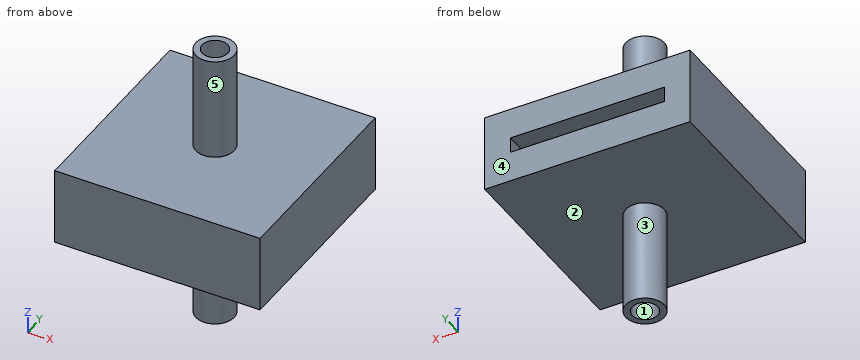
from build123d import *

# Parameters (mm, degrees)
F0_W      = 50.8
F0_H      = 50.8
F1_DEPTH  = 19.05
F2_W      = 38.1
F2_H      = 3.81
F3_DEPTH  = 38.1
F5_R      = 4.7625
F6_DEPTH  = 25.4
F7_R      = 4.7625
F8_DEPTH  = 25.4
F9_R      = 3.175
F10_DEPTH = 74.676


with BuildPart() as f1:
    # F0 (on Top) → F1 (new body)
    with BuildSketch(Plane.XY):
        Rectangle(F0_W, F0_H)
    extrude(amount=F1_DEPTH)

    # F2 (on face) → F3 (cut)
    with BuildSketch(Plane(origin=(0, 25.4, 0), x_dir=(-1, 0, 0), z_dir=(0, 1, 0))):
        with Locations((0, 9.525)):
            Rectangle(F2_W, F2_H)
    extrude(amount=-F3_DEPTH, mode=Mode.SUBTRACT)

    # F5 (on face) → F6 (join)
    with BuildSketch(Plane.XY.offset(19.05)):
        Circle(F5_R)
    extrude(amount=F6_DEPTH)

    # F7 (on face) → F8 (join)
    with BuildSketch(Plane(origin=(0, 0, 0), x_dir=(1, 0, 0), z_dir=(0, 0, -1))):
        Circle(F7_R)
    extrude(amount=F8_DEPTH)

    # F9 (on face) → F10 (cut)
    with BuildSketch(Plane(origin=(0, 0, -25.4), x_dir=(1, 0, 0), z_dir=(0, 0, -1))):
        Circle(F9_R)
    extrude(amount=-F10_DEPTH, mode=Mode.SUBTRACT)


solid = f1.part
The model under review builds one solid part; all positions refer to its coordinate system, in mm. Face numbers are marked on the shaded views. A direction names the side the tool comes from. Round coordinates to 2 decimals unless told otherwise and drop trailing zeros. Write each loop counter-clockwise with the first axis right and the second up, starting at its lowest first coordinate (ties: lowest second). Pieces come first, ordered by that corner, then holes. Notation, with made-up numbers: (15, 29) - (30, 29) arc R28 ccw to (30, 57) - close; hole circle Ø5 at (20, 74). An arc over 180 degrees is marked (long way). One line per item, written item: value. Start each with the question number.
1. To check wall thickness, follow L1, parallel to Z at x = 16, y = 20.5; L2, parallel to Y at x = 0, z = 24 (1 decimal). State the ranges of each line that lie inside material, in increasing order. Write a range as from..to.
2. The part is to be moulded in two halves that separate along Y. For the marked faces 1, 2 and 3, say which applies: released by +Y, released by -Y, zero draft, split by the parting line, or undercut.
3. Clearance check with flat-ended pins moving along their axes: P1, Ø2, axis at x = 7, z = 28, coming from the -Y side; P2, Ø1.5, axis at x = -5, z = 21, coming from the -Y side; P3, Ø4, axis at x = 13, y = 16.5, coming from the +Z side. State where each tip first meets the part, or that it passes through.
4. Consider section C-C on x = -18. Write out the cut boundary in (y, z), and give its area (3 significant figures).
5. Consider section D-D on y = -8. Write out the cut boundary in (x, z).
6. Machinability: for the marked faces 4 and 5, which of the approach directions +Z, -Z, +X, -X, +Y, -Y give a long, thin tool a straight path to every point of the face, cutting with its end or side? Answer none if there is none.
7. Consider section B-B on x = 0. State how many separate pieces and enclosed holes the cut face has, and give its area (3 significant figures).
Checks:
1. L1: z = 0..7.62, 11.43..19.05
1. L2: y = -4.8..-3.2, 3.2..4.8
2. face 1: undercut
2. face 2: zero draft
2. face 3: split by the parting line
3. P1: passes through
3. P2: stops at y = -2.15
3. P3: stops at z = 19.05
4. outline: (-25.4, 0) - (25.4, 0) - (25.4, 7.62) - (-12.7, 7.62) - (-12.7, 11.43) - (25.4, 11.43) - (25.4, 19.05) - (-25.4, 19.05) - close
4. area: 823 mm^2
5. outline: (-25.4, 0) - (25.4, 0) - (25.4, 19.05) - (-25.4, 19.05) - close; hole (-19.05, 7.62) - (19.05, 7.62) - (19.05, 11.43) - (-19.05, 11.43) - close
6. face 4: +Z, -Z, +X, -X, +Y
6. face 5: +Z
7. separate pieces: 3
7. enclosed holes: 0
7. area: 887 mm^2
